Design review of the part shown in the three views and the two pictorial views. Dimensions are in mm from the part's minimum x, y and z. A direction names the side the tool comes from. Give positions to 0.01 mm unless a question says otherwise; leave off trailing zeros. Loops run counter-clockwise (first coordinate to the right, second up) from the corner with the lowest first, then second, coordinate; pieces in that order, holes last. Notation, with made-up numbers: (-30.5, 66.25) - (-2.5, 66.25) arc R20 cw to (-2.5, 93.25) - close; hole circle Ø9 at (31.25, 43.25). An arc over 180 degrees is marked (long way). Answer in a Markdown table with one row per item.
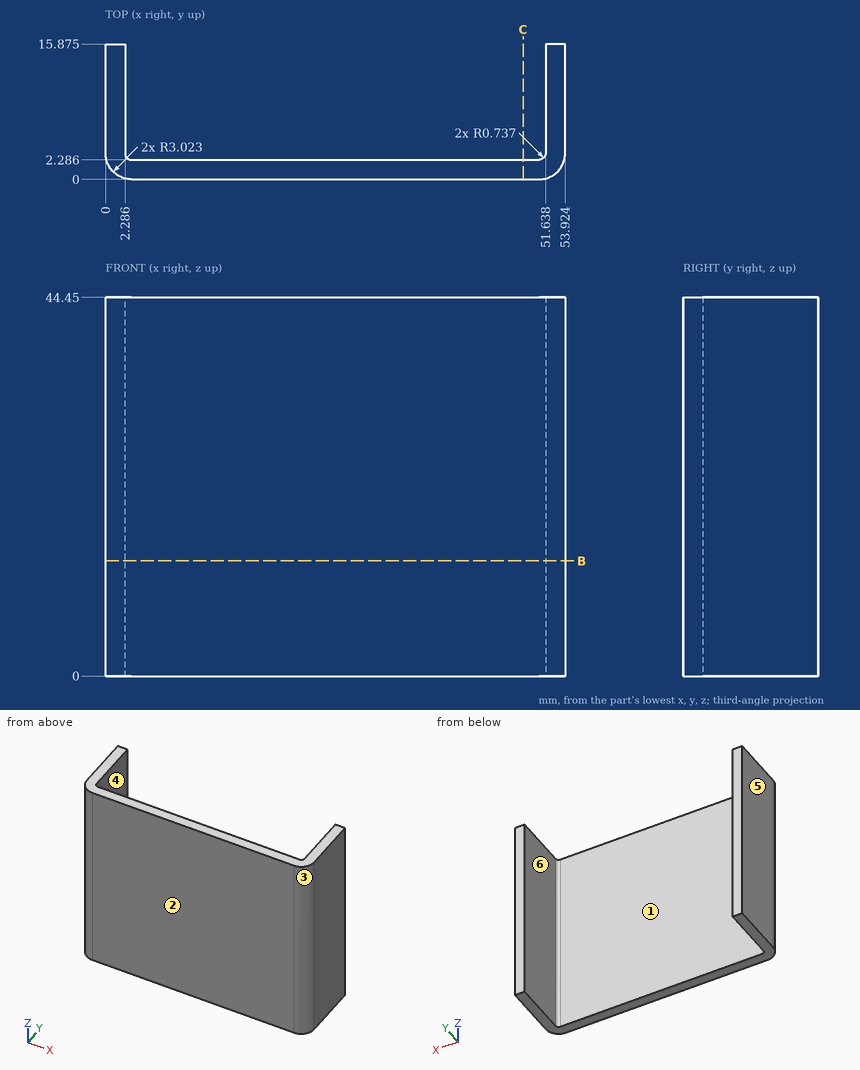
1. For the marked faces 5 and 6, list the 3-axis set-ups (+Z, -Z, +X, -X, +Y, -Y) from which the entire face can be reached by the end or side of a thin tool; tool diameter is ignored.
Values:
| item | result |
|---|---|
| face 5 | +Z, -Z, -X, +Y, -Y |
| face 6 | +Z, -Z, +Y |
2. Mouldability with a two-part tool opening along X and no side actions: class the marked faces 1, 2, 3 and 4 as released by +X, released by -X, zero draft, split by the parting line, or undercut.
Values:
| item | result |
|---|---|
| face 1 | undercut |
| face 2 | zero draft |
| face 3 | released by +X |
| face 4 | undercut |
3. Clearance check with flat-ended pins moving along their axes: pin 1 (6 mm diameter, centred on x = 13, y = 6.5, fed in from +Z); pin 2 (4 mm diameter, centred on x = 24.5, z = 15.5, fed in from +Y). State where each tip first meets the part, or that it passes through.
Values:
| item | result |
|---|---|
| pin 1 | passes through |
| pin 2 | stops at y = 2.29 |
4. We need section C-C, the plane x = 49. Give the boundary of the cut face in (y, z).
Values:
| item | result |
|---|---|
| outline | (0, 0) - (2.29, 0) - (2.29, 44.45) - (0, 44.45) - close |
5. We need section B-B, the plane z = 13.5. Give the boundary of the cut face in (x, y) (1 decimal).
Values:
| item | result |
|---|---|
| outline | (0, 3) arc R3 ccw to (3, 0) - (50.9, 0) arc R3 ccw to (53.9, 3) - (53.9, 15.9) - (51.6, 15.9) - (51.6, 3) arc R0.7 cw to (50.9, 2.3) - (3, 2.3) arc R0.7 cw to (2.3, 3) - (2.3, 15.9) - (0, 15.9) - close |
6. Wall thickness on line 1 (X direction, y = 9.5, z = 26) (1 decimal); line 2 (Y direction, x = 18.5, z = 35.5); line 3 (X direction, y = 2.5, z = 22) (1 decimal): over which ranges is each line inside the solid? List them lowest first. Write a range as [from, to].
Values:
| item | result |
|---|---|
| line 1 | x = [0, 2.3], [51.6, 53.9] |
| line 2 | y = [0, 2.29] |
| line 3 | x = [0, 2.5], [51.4, 53.9] |
